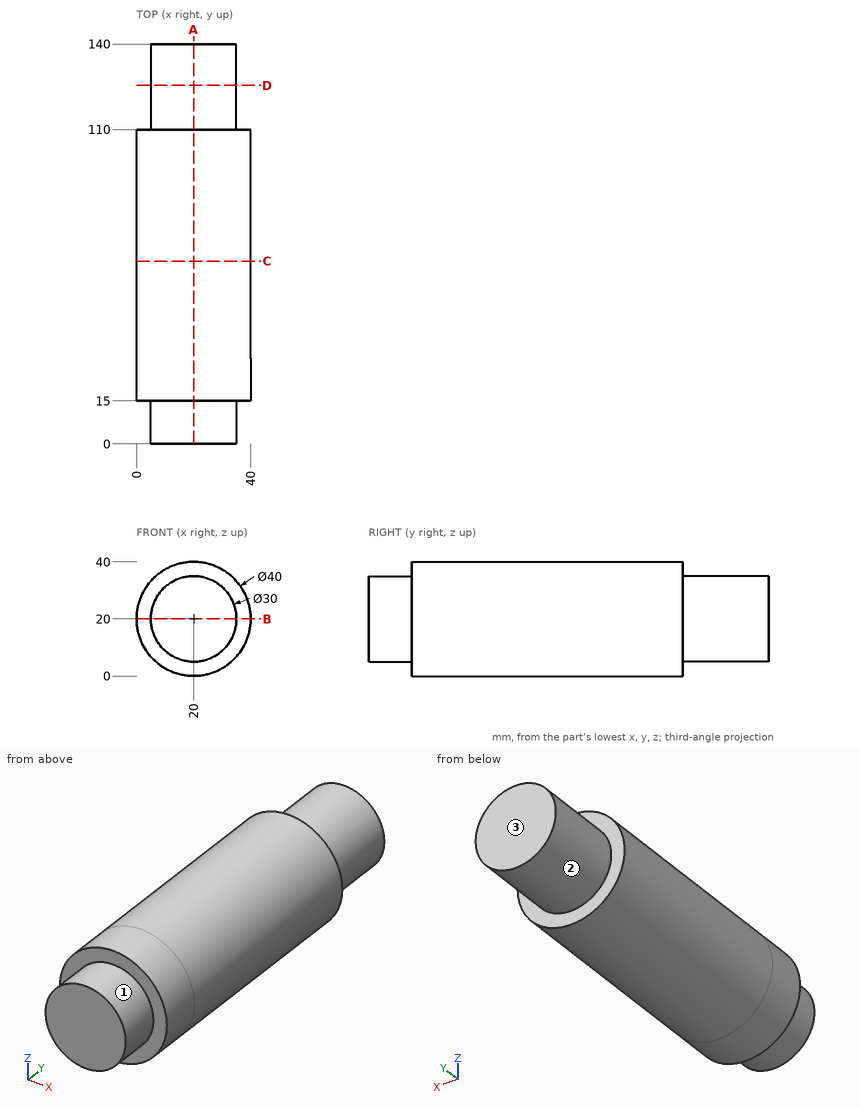
The figure shows three views and two pictorial views of one solid part (mm, origin at its lowest corner). Answer the questions. A direction names the side the tool comes from. Coordinates: 2 decimals unless noted, no trailing zeros. Loops run counter-clockwise (first coordinate to the right, second up) from the corner with the lowest first, then second, coordinate; pieces in that order, holes last.
1) A tool of negligible diameter and unlimited length cuts with its end or side. For the marked faces 1, 2 and 3, from which of +Z, -Z, +X, -X, +Y, -Y can it reach the whole face along a straight path? Write none if from no direction.
2) Find section D-D on y = 125.5. Write down the section's boundary in (x, z).
3) Find section C-C on y = 64. Write down the section's boundary in (x, z).
4) Find section B-B on z = 20. Write down the section's boundary in (x, y), then the cut area to 3 significant figures.
5) Find section A-A on x = 20. Write down the section's boundary in (y, z).
6) Find the intervals of material crossed by L1, parallel to X at y = 105, z = 19; L2, parallel to Z at x = 20, y = 125.5; L3, parallel to Y at x = 23.5, z = 3, in increasing order.
7) Flat-ended cylindrical pins translate along their axes: pin 1 Ø1.5 at (x, y) = (23, 114.5) entering from +Z; pin 2 Ø3 at (y, z) = (26, 30.5) entering from -X; pin 3 Ø4 at (x, y) = (17, 41) entering from +Z (3 decimals); pin 4 Ø12 at (x, z) = (23.5, 28.5) entering from -Y. Find the tip coordinate at first contact, or state that the pin passes through.
Values:
1. face 1: -Y
1. face 2: +Y
1. face 3: +Z, -Z, +X, -X, +Y
2. outline: circle Ø30 at (20, 20)
3. outline: circle Ø40 at (20, 20)
4. outline: (0, 15) - (5, 15) - (5, 0) - (35, 0) - (35, 15) - (40, 15) - (40, 110) - (35, 110) - (35, 140) - (5, 140) - (5, 110) - (0, 110) - close
4. area: 5,150 mm2
5. outline: (0, 5) - (15, 5) - (15, 0) - (110, 0) - (110, 5) - (140, 5) - (140, 35) - (110, 35) - (110, 40) - (15, 40) - (15, 35) - (0, 35) - close
6. L1: x = 0.03 to 39.97
6. L2: z = 5 to 35
6. L3: y = 15 to 110
7. pin 1: stops at z = 34.83
7. pin 2: stops at x = 2.14
7. pin 3: stops at z = 39.975
7. pin 4: stops at y = 0
